```python
from build123d import *

# Parameters (mm, degrees)
F1_DEPTH = 100
F3_DEPTH = 50
F5_DEPTH = 300
F6_R     = 100
F7_DEPTH = 450.001


with BuildPart() as f1:
    # F0 (on Top) → F1 (new body)
    with BuildSketch(Plane.XY):
        with BuildLine():
            ThreePointArc((-595, 300), (-895, 0), (-595, -300))
            Line((-595, -300), (495, -300))
            ThreePointArc((495, -300), (565.710678, -270.710678), (595, -200))
            Line((595, -200), (595, 200))
            ThreePointArc((595, 200), (565.710678, 270.710678), (495, 300))
            Line((495, 300), (-595, 300))
        make_face()
    extrude(amount=F1_DEPTH)

    # F2 (on face) → F3 (join)
    with BuildSketch(Plane(origin=(0, 0, 0), x_dir=(1, 0, 0), z_dir=(0, 0, -1))):
        with BuildLine():
            ThreePointArc((-595, 300), (-717.474487, 273.861279), (-818.606798, 200))
            Line((-818.606798, 200), (-307.265759, 200))
            Line((-307.265759, 200), (-307.265759, 300))
            Line((-307.265759, 300), (-595, 300))
        make_face()
        with BuildLine():
            Line((-307.265759, -200), (-818.606798, -200))
            ThreePointArc((-818.606798, -200), (-717.474487, -273.861279), (-595, -300))
            Line((-595, -300), (-307.265759, -300))
            Line((-307.265759, -300), (-307.265759, -200))
        make_face()
    extrude(amount=F3_DEPTH)

    # F4 (on face) → F5 (join)
    with BuildSketch(Plane.XY.offset(100)):
        with BuildLine():
            ThreePointArc((-407.65006, -70), (-398.187922, -35.566923), (-395, 0))
            ThreePointArc((-395, 0), (-398.187922, 35.566923), (-407.65006, 70))
            ThreePointArc((-407.65006, 70), (-447.1271, 134.661076), (-507.822021, 180))
            ThreePointArc((-507.822021, 180), (-795, 0), (-507.822021, -180))
            ThreePointArc((-507.822021, -180), (-447.1271, -134.661076), (-407.65006, -70))
        make_face()
    extrude(amount=F5_DEPTH)

    # F6 (on face) → F7 (cut, through all)
    with BuildSketch(Plane.XY.offset(400)):
        with Locations((-595, 0)):
            Circle(F6_R)
    extrude(amount=-F7_DEPTH, mode=Mode.SUBTRACT)


solid = f1.part
```
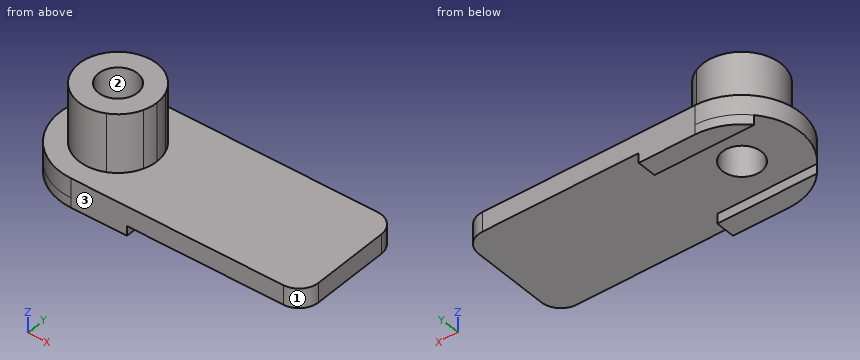
Check sheet for the modelled part. Datum: model origin and axes. Units: mm. Face numbers are marked on the shaded views. Round coordinates to 2 decimals unless told otherwise and drop trailing zeros. Write each loop counter-clockwise with the first axis right and the second up, starting at its lowest first coordinate (ties: lowest second). Pieces come first, ordered by that corner, then holes. Notation, with made-up numbers: (43.25, 83.25) -> (86.25, 83.25) arc R16 cw to (86.25, 97.25) -> close; hole circle Ø2 at (-31, -17.75). An arc over 180 degrees is marked (long way). Put each result on its own line as item: value.
(1) Sectioned sample at A-A (x = -619). Enter the section's corners in (y, z), plus the area to 3 significant figures.
Values found:
outline: (-299.04, -50) -> (-200, -50) -> (-200, 0) -> (-97.08, 0) -> (-97.08, 400) -> (-198.55, 400) -> (-198.55, 100) -> (-299.04, 100) -> close; (97.08, 0) -> (200, 0) -> (200, -50) -> (299.04, -50) -> (299.04, 100) -> (198.55, 100) -> (198.55, 400) -> (97.08, 400) -> close
area: 111,000 mm^2
(2) Sectioned sample at C-C (y = -256). Enter the section's corners in (x, z), plus the area to 3 significant figures.
Values found:
outline: (-751.41, -50) -> (-307.27, -50) -> (-307.27, 0) -> (577.85, 0) -> (577.85, 100) -> (-751.41, 100) -> close
area: 155,000 mm^2
(3) Sectioned sample at B-B (z = 217.5). Enter the section's corners in (x, y).
Values found:
outline: (-507.82, -180) arc R200 ccw to (-407.65, -70) arc R200 ccw to (-395, 0) arc R200 ccw to (-407.65, 70) arc R200 ccw to (-507.82, 180) arc R200 ccw (long way) to start; hole circle Ø200 at (-595, 0)
(4) Sectioned sample at D-D (x = -275.5). Enter the section's corners in (y, z), plus the area to 3 significant figures.
Values found:
outline: (-300, 0) -> (300, 0) -> (300, 100) -> (-300, 100) -> close
area: 60,000 mm^2
(5) Mould release check, pull along X, two halves, no side actions. Record for the marked faces 1, 2 and 3: released by +X, released by -X, zero draft, split by the parting line, or undercut.
Values found:
face 1: released by +X
face 2: undercut
face 3: zero draft
(6) Material ranges on line 1 (Y direction, x = -595, z = 226); line 2 (Y direction, x = -600, z = 339); line 3 (Z direction, x = 382, y = 199), recorded low to high.
Values found:
line 1: y = -200 to -100, 100 to 200
line 2: y = -199.94 to -99.87, 99.87 to 199.94
line 3: z = 0 to 100
(7) Go/stop test with flat-tipped pins: pin 1 Ø10 at (y, z) = (-26, 97) entering from -X; pin 2 Ø5 at (y, z) = (-22.5, 292.5) entering from -X; pin 3 Ø6 at (x, y) = (-385.5, -104) entering from +Z. Record where each tip stops, or that it passes through.
Values found:
pin 1: stops at x = -894.26
pin 2: stops at x = -794
pin 3: stops at z = 100
